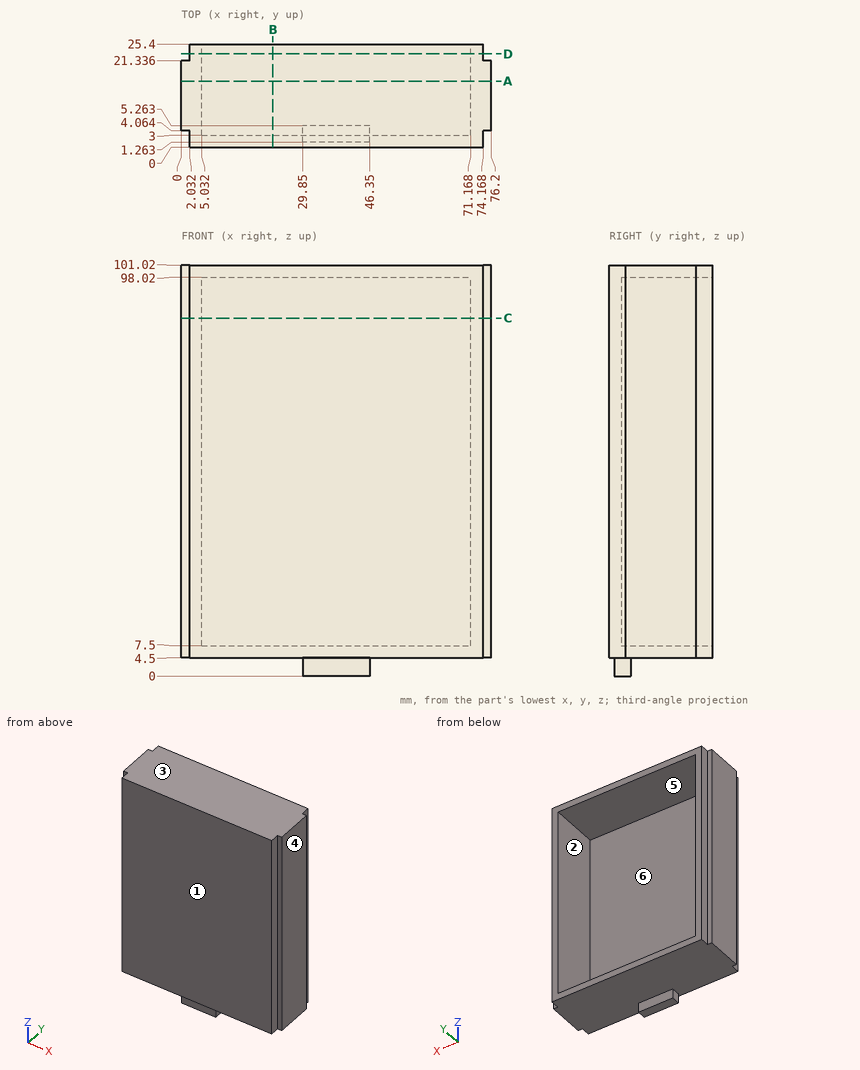
Verification items for this drawing (mm, ordinates from the low corner). A direction names the side the tool comes from. Coordinates: 2 decimals unless noted, no trailing zeros. Loops run counter-clockwise (first coordinate to the right, second up) from the corner with the lowest first, then second, coordinate; pieces in that order, holes last. Notation, with made-up numbers: (-11, 15) -> (47, 15) arc R29 cw to (47, 44) -> close; hole circle Ø4 at (60, 26). An arc over 180 degrees is marked (long way). Answer in a Markdown table with one row per item. Add a question column.
1. Section check C-C, the plane z = 88. Enter the section's corners in (x, y), then the cut area to 3 significant figures.
2. Section check A-A, the plane y = 16.25. Enter the section's corners in (x, z).
3. Material ranges on probe 1 along Z at (x, y) = (40.5, 3.25); probe 2 along X at (y, z) = (11.75, 15); probe 3 along Z at (x, y) = (23, 18.25), recorded low to high. Write a range as [from, to].
4. Section check D-D, the plane y = 23. Enter the section's corners in (x, z).
5. Draft check along Z on the marked faces 3, 4, 5 and 6. Enter one of: +Z half, -Z half, draft (parallel to the pull), parting line (faces both ways), or undercut.
6. Section check B-B, the plane x = 22.5. Enter the section's corners in (y, z).
7. Depth check by flat-ended pin: P1, Ø12.5, axis at x = 56, y = 8.5, coming from the -Z side; P2, Ø1, axis at x = 68, z = 31, coming from the +Y side; P3, Ø3.5, axis at x = 37.5, z = 2, coming from the +Y side. Enter the tip coordinate at first touch or a pass-through.
8. Access from +Z, -Z, +X, -X, +Y, -Y to the whole of each face (thin tool, end or side, straight path). Record for the marked faces 1 and 2.
Derived:
| question | item | result |
|---|---|---|
| 1 | outline | (0, 4.06) -> (2.03, 4.06) -> (2.03, 0) -> (74.17, 0) -> (74.17, 4.06) -> (76.2, 4.06) -> (76.2, 21.34) -> (74.17, 21.34) -> (74.17, 25.4) -> (71.17, 25.4) -> (71.17, 3) -> (5.03, 3) -> (5.03, 25.4) -> (2.03, 25.4) -> (2.03, 21.34) -> (0, 21.34) -> close |
| 1 | area | 421 mm² |
| 2 | outline | (0, 4.5) -> (76.2, 4.5) -> (76.2, 101.02) -> (0, 101.02) -> close; hole (5.03, 7.5) -> (71.17, 7.5) -> (71.17, 98.02) -> (5.03, 98.02) -> close |
| 3 | probe 1 | z = [0, 7.5], [98.02, 101.02] |
| 3 | probe 2 | x = [0, 5.03], [71.17, 76.2] |
| 3 | probe 3 | z = [4.5, 7.5], [98.02, 101.02] |
| 4 | outline | (2.03, 4.5) -> (74.17, 4.5) -> (74.17, 101.02) -> (2.03, 101.02) -> close; hole (5.03, 7.5) -> (71.17, 7.5) -> (71.17, 98.02) -> (5.03, 98.02) -> close |
| 5 | face 3 | +Z half |
| 5 | face 4 | draft |
| 5 | face 5 | undercut |
| 5 | face 6 | undercut |
| 6 | outline | (0, 4.5) -> (25.4, 4.5) -> (25.4, 7.5) -> (3, 7.5) -> (3, 98.02) -> (25.4, 98.02) -> (25.4, 101.02) -> (0, 101.02) -> close |
| 7 | P1 | stops at z = 4.5 |
| 7 | P2 | stops at y = 3 |
| 7 | P3 | stops at y = 5.26 |
| 8 | face 1 | +Z, -Z, +X, -X, -Y |
| 8 | face 2 | +Y |
